from build123d import *

# Parameters (mm, degrees)
SKETCH1_W                    = 15
SKETCH1_H                    = 15
BOSS_EXTRUDE1_DEPTH          = 261
SKETCH2_W                    = 13
SKETCH2_H                    = 13
CUT_EXTRUDE1_DEPTH           = 261
F_3_0_3_DIAMETER_HOLE1_D     = 3
F_3_0_3_DIAMETER_HOLE2_D     = 3
F_6_0_6_DIAMETER_HOLE1_D     = 6
F_6_0_6_DIAMETER_HOLE1_DEPTH = 10
F_6_0_6_DIAMETER_HOLE1_TIP   = 1.802581857
F_3_0_3_DIAMETER_HOLE3_D     = 3


with BuildPart() as part:
    # Sketch1 → Boss-Extrude1 (new body)
    with BuildSketch(Plane.XY):
        with Locations((-36.796141786, 14.648070893)):
            Rectangle(SKETCH1_W, SKETCH1_H)
    extrude(amount=BOSS_EXTRUDE1_DEPTH)

    # Sketch2 → Cut-Extrude1 (cut)
    with BuildSketch(Plane(origin=(0, 0, 0), x_dir=(-1, 0, 0), z_dir=(0, 0, -1))):
        with Locations((36.796141786, 14.648070893)):
            Rectangle(SKETCH2_W, SKETCH2_H)
    extrude(amount=-CUT_EXTRUDE1_DEPTH, mode=Mode.SUBTRACT)

    # Ø3.0 (3) Diameter Hole1 (through all)
    with Locations(Plane(origin=(0, 22.148070893, 0), x_dir=(1, 0, 0), z_dir=(0, 1, 0))):
        with Locations((-36.796141786, -256), (-36.796141786, -231)):
            Hole(F_3_0_3_DIAMETER_HOLE1_D / 2)

    # Ø3.0 (3) Diameter Hole2 (through all)
    with Locations(Plane(origin=(0, 22.148070893, 0), x_dir=(1, 0, 0), z_dir=(0, 1, 0))):
        with Locations((-36.796141786, -12), (-36.796141786, -28)):
            Hole(F_3_0_3_DIAMETER_HOLE2_D / 2)

    # Ø6.0 (6) Diameter Hole1
    with Locations(Plane(origin=(0, 22.148070893, 0), x_dir=(1, 0, 0), z_dir=(0, 1, 0))):
        with Locations((-36.796141786, -20)):
            Hole(F_6_0_6_DIAMETER_HOLE1_D / 2, depth=F_6_0_6_DIAMETER_HOLE1_DEPTH)
            with Locations((0, 0, -(F_6_0_6_DIAMETER_HOLE1_DEPTH + F_6_0_6_DIAMETER_HOLE1_TIP / 2))):  # 118° drill point
                Cone(0, F_6_0_6_DIAMETER_HOLE1_D / 2, F_6_0_6_DIAMETER_HOLE1_TIP, mode=Mode.SUBTRACT)

    # Ø3.0 (3) Diameter Hole3 (through all)
    with Locations(Plane.ZY.offset(44.296141786)):
        with Locations((16, 14.648070893)):
            Hole(F_3_0_3_DIAMETER_HOLE3_D / 2)


solid = part.part
Geometry check sheet. Reference: the model listing, model coordinates, mm. A direction names the side the tool comes from. Give positions to 0.01 mm unless a question says otherwise; leave off trailing zeros. Write each loop counter-clockwise with the first axis right and the second up, starting at its lowest first coordinate (ties: lowest second). Pieces come first, ordered by that corner, then holes.
1) Go/stop test with flat-tipped pins: pin 1 Ø1.8 at (x, z) = (-36.8, 256) entering from +Y; pin 2 Ø4 at (x, z) = (-36.8, 231) entering from -Y; pin 3 Ø5 at (x, z) = (-36.8, 20) entering from +Y. Record where each tip stops, or that it passes through.
Values follow:
pin 1: passes through
pin 2: stops at y = 7.15
pin 3: stops at y = 8.15
2) Cross-section at A-A (y = 11). Record the boundary of the cut face in (x, z).
Values follow:
outline: (-44.3, 0) - (-43.3, 0) - (-43.3, 261) - (-44.3, 261) - close; (-30.3, 0) - (-29.3, 0) - (-29.3, 261) - (-30.3, 261) - close
3) Set-up check for faces 1 (the face through (-39.567, 21.641, 21.149)), 2 (the face through (-29.296, 15, 129)), 3 (the face through (-30.296, 15, 129)): record each of +Z, -Z, +X, -X, +Y, -Y from which the full face is reachable in a straight line by a thin tool's end or side.
Values follow:
face 1: +Y
face 2: +Z, -Z, +X, +Y, -Y
face 3: +Z, -Z
4) Release check for a two-part mould opening along Y. For faces 4 (the face through (-44, 15, 261)), 5 (the face through (-37, 7.148, 129)), 6 (the face through (-43.296, 15, 129)) record: released by +Y, released by -Y, zero draft, split by the parting line, or undercut.
Values follow:
face 4: zero draft
face 5: released by -Y
face 6: undercut
5) Thickness scan on line 1 (X direction, y = 15.25, z = 106); line 2 (Y direction, x = -40, z = 93.5); line 3 (X direction, y = 7.55, z = 28). Record the ranges inside material, lowest first.
Values follow:
line 1: x = -44.3 to -43.3, -30.3 to -29.3
line 2: y = 7.15 to 8.15, 21.15 to 22.15
line 3: x = -44.3 to -38.3, -35.3 to -29.3
6) Cross-section at C-C (z = 71). Record the boundary of the cut face in (x, y).
Values follow:
outline: (-44.3, 7.15) - (-29.3, 7.15) - (-29.3, 22.15) - (-44.3, 22.15) - close; hole (-43.3, 8.15) - (-30.3, 8.15) - (-30.3, 21.15) - (-43.3, 21.15) - close
7) Cross-section at B-B (z = 20). Record the boundary of the cut face in (x, y).
Values follow:
outline: (-44.3, 7.15) - (-29.3, 7.15) - (-29.3, 22.15) - (-33.8, 22.15) - (-33.8, 21.15) - (-30.3, 21.15) - (-30.3, 8.15) - (-43.3, 8.15) - (-43.3, 21.15) - (-39.8, 21.15) - (-39.8, 22.15) - (-44.3, 22.15) - close
